```python
from build123d import *

# Parameters (mm, degrees)
FILLET1_R = 0.508


with BuildPart() as part:
    # Sketch1 → Revolve1 (revolve)
    with BuildSketch(Plane.XY):
        Polygon((0, 0), (0, 3.81), (50.8, 3.81), (50.8, 0), (37.892541774, 0), (12.907458226, 0), align=None)
    revolve(axis=Axis((0, 3.81, 0), (1, 0, 0)))

    # Sketch6 → Tap Drill for M4 Helicoil1 (revolve, cut)
    with BuildSketch(Plane.ZX.offset(3.81)):
        Polygon((0, 0), (0, 10.1518073), (2.1, 8.89), (2.1, 0), align=None)
    tap_drill_for_m4_helicoil1 = revolve(axis=Axis((-6.35, 3.81, 0), (1, 0, 0)), mode=Mode.SUBTRACT)

    # Mirror1: Tap Drill for M4 Helicoil1 across plane
    add(tap_drill_for_m4_helicoil1.mirror(Plane.ZY.offset(-25.4)), mode=Mode.SUBTRACT)

    # Fillet1
    fillet1_edges = [part.edges().sort_by_distance(p)[0] for p in [
        (0, 3.81, -2.1),
        (50.8, 3.81, -2.1),
    ]]
    fillet(fillet1_edges, radius=FILLET1_R)


solid = part.part
```
Verification items for the finished model (mm, model axes). A direction names the side the tool comes from. Give positions to 0.01 mm unless a question says otherwise; leave off trailing zeros. Order: outer loops, then holes, each group sorted by start corner. A loop starts at its lowest first (then second) coordinate and runs counter-clockwise, first axis right, second up. Notation, with made-up numbers: (39, 58) -> (79, 58) arc R20 cw to (79, 93) -> close; hole circle Ø6 at (-0.5, 78.25). An arc over 180 degrees is marked (long way). Use a Markdown table: item, result.
1) Mould release check, pull along Z, two halves, no side actions. Record for faces 3 (the flat face through (50.8, 5.4, 2.5)), 4 (the cylindrical face through (25.76, 6.83, 2.32)), 5 (the cylindrical face through (46.16, 1.728, -0.273)): pulls with the +Z half, pulls with the -Z half, needs draft (parallel to the pull), parting line crosses it, or undercut.
Results:
| item | result |
|---|---|
| face 3 | needs draft |
| face 4 | parting line crosses it |
| face 5 | undercut |
2) Material ranges on probe 1 along Y at (x, z) = (4.5, 0); probe 2 along Z at (x, y) = (45, 3.81); probe 3 along Y at (x, z) = (9, 1.25), recorded low to high.
Results:
| item | result |
|---|---|
| probe 1 | 0 to 1.71, 5.91 to 7.62 |
| probe 2 | -3.81 to -2.1, 2.1 to 3.81 |
| probe 3 | 0.21 to 2.36, 5.26 to 7.41 |
3) Section check A-A, the plane x = 43.5. Record the boundary of the cut face in (y, z), then the cut area to 3 significant figures.
Results:
| item | result |
|---|---|
| outline | circle Ø7.62 at (3.81, 0); hole circle Ø4.2 at (3.81, 0) |
| area | 31.7 mm² |
4) Section check C-C, the plane y = 7. Record the boundary of the cut face in (x, z).
Results:
| item | result |
|---|---|
| outline | (0, -2.08) -> (50.8, -2.08) -> (50.8, 2.08) -> (0, 2.08) -> close |
5) Tool access check on faces 1 (the cylindrical face through (4.64, 1.728, -0.273)), 2 (the flat face through (0, 1, 1)). Record the directions out of +Z, -Z, +X, -X, +Y, -Y that give a thin tool (end or side, any length) a straight path to the whole face; none if there is none.
Results:
| item | result |
|---|---|
| face 1 | -X |
| face 2 | +Z, -Z, -X, +Y, -Y |
6) Depth check by flat-ended pin: pin 1 Ø2.5 at (y, z) = (3.81, 0) entering from -X; pin 2 Ø3 at (x, y) = (30, 5.5) entering from +Z; pin 3 Ø1.5 at (x, z) = (25.5, -1) entering from -Y. Enter the tip coordinate at first touch or a pass-through.
Results:
| item | result |
|---|---|
| pin 1 | x = 9.4 |
| pin 2 | z = 3.81 |
| pin 3 | y = 0.01 |
7) Section check B-B, the plane x = 27. Record the boundary of the cut face in (y, z), then the cut area to 3 significant figures.
Results:
| item | result |
|---|---|
| outline | circle Ø7.62 at (3.81, 0) |
| area | 45.6 mm² |
